```python
from build123d import *

# Parameters (mm, degrees)
SKETCH1_R           = 140
SKETCH1_R_2         = 5
SKETCH1_R_3         = 2.5
BOSS_EXTRUDE1_DEPTH = 2


with BuildPart() as part:
    # Sketch1 → Boss-Extrude1 (new body)
    with BuildSketch(Plane(origin=(0, 0, 0), x_dir=(1, 0, 0), z_dir=(0, 1, 0))):
        with Locations(Location((0, 0, 0), (0, 0, 270))):
            Circle(SKETCH1_R)
        with Locations(Location((-99.592921435, 57.5, 0), (0, 0, 270))):
            Circle(SKETCH1_R_2, mode=Mode.SUBTRACT)
        with Locations(Location((-57.5, 99.592921435, 0), (0, 0, 270))):
            Circle(SKETCH1_R_2, mode=Mode.SUBTRACT)
        with Locations(Location((57.5, 99.592921435, 0), (0, 0, 90))):
            Circle(SKETCH1_R_2, mode=Mode.SUBTRACT)
        with Locations(Location((99.592921435, 57.5, 0), (0, 0, 90))):
            Circle(SKETCH1_R_2, mode=Mode.SUBTRACT)
        with Locations(Location((99.592921435, -57.5, 0), (0, 0, 270))):
            Circle(SKETCH1_R_2, mode=Mode.SUBTRACT)
        with Locations(Location((57.5, -99.592921435, 0), (0, 0, 270))):
            Circle(SKETCH1_R_2, mode=Mode.SUBTRACT)
        with Locations(Location((-57.5, -99.592921435, 0), (0, 0, 90))):
            Circle(SKETCH1_R_2, mode=Mode.SUBTRACT)
        with Locations(Location((-99.592921435, -57.5, 0), (0, 0, 90))):
            Circle(SKETCH1_R_2, mode=Mode.SUBTRACT)
        with Locations(Location((0, 115, 0), (0, 0, 270))):
            Circle(SKETCH1_R_2, mode=Mode.SUBTRACT)
        with Locations(Location((0, -115, 0), (0, 0, 90))):
            Circle(SKETCH1_R_2, mode=Mode.SUBTRACT)
        with Locations(Location((-115, 0, 0), (0, 0, 270))):
            Circle(SKETCH1_R_2, mode=Mode.SUBTRACT)
        with Locations(Location((115, 0, 0), (0, 0, 90))):
            Circle(SKETCH1_R_2, mode=Mode.SUBTRACT)
        with Locations(Location((-10.352761804, 38.637033052, 0), (0, 0, 270))):
            Circle(SKETCH1_R_3, mode=Mode.SUBTRACT)
        with Locations(Location((-28.284271247, 28.284271247, 0), (0, 0, 270))):
            Circle(SKETCH1_R_3, mode=Mode.SUBTRACT)
        with Locations(Location((-38.637033052, 10.352761804, 0), (0, 0, 270))):
            Circle(SKETCH1_R_3, mode=Mode.SUBTRACT)
        with Locations(Location((-38.637033052, -10.352761804, 0), (0, 0, 270))):
            Circle(SKETCH1_R_3, mode=Mode.SUBTRACT)
        with Locations(Location((38.637033052, -10.352761804, 0), (0, 0, 90))):
            Circle(SKETCH1_R_3, mode=Mode.SUBTRACT)
        with Locations(Location((38.637033052, 10.352761804, 0), (0, 0, 90))):
            Circle(SKETCH1_R_3, mode=Mode.SUBTRACT)
        with Locations(Location((28.284271247, 28.284271247, 0), (0, 0, 90))):
            Circle(SKETCH1_R_3, mode=Mode.SUBTRACT)
        with Locations(Location((10.352761804, 38.637033052, 0), (0, 0, 90))):
            Circle(SKETCH1_R_3, mode=Mode.SUBTRACT)
        with Locations(Location((28.284271247, -28.284271247, 0), (0, 0, 270))):
            Circle(SKETCH1_R_3, mode=Mode.SUBTRACT)
        with Locations(Location((-28.284271247, -28.284271247, 0), (0, 0, 90))):
            Circle(SKETCH1_R_3, mode=Mode.SUBTRACT)
        with Locations(Location((10.352761804, -38.637033052, 0), (0, 0, 270))):
            Circle(SKETCH1_R_3, mode=Mode.SUBTRACT)
        with Locations(Location((-10.352761804, -38.637033052, 0), (0, 0, 90))):
            Circle(SKETCH1_R_3, mode=Mode.SUBTRACT)
    extrude(amount=BOSS_EXTRUDE1_DEPTH)


solid = part.part
```
The listing builds one solid part. Answer for the finished solid, in the listing's coordinates (mm). Round coordinates to 2 decimals unless told otherwise and drop trailing zeros. Loops run counter-clockwise (first coordinate to the right, second up) from the corner with the lowest first, then second, coordinate; pieces in that order, holes last. Notation, with made-up numbers: (-28, -19.5) - (3, -19.5) arc R15 cw to (3, -12.5) - close; hole circle Ø7 at (11.25, 19.5). An arc over 180 degrees is marked (long way). Use one line per item in the form item = value. Start each with the question number.
1. For a pull along X with two mould halves and no side action, classify faces 1 (the face through (2, 2, -2)), 2 (the face through (-85.19, 0.99, -111.1)), 3 (the face through (-96.214, 0.986, -61.185)) as pulls with the +X half, pulls with the -X half, needs draft (parallel to the pull), parting line crosses it, or undercut.
2. The part is cut by section C-C on z = -115. Determine the outline of the cut face in (x, y), then the cut area to 3 significant figures.
3. Consider line 1 (X direction, y = 0.55, z = 0); line 2 (X direction, y = 1.7, z = -104); line 3 (Z direction, x = -100.5, y = 1.15). Determine where each line is inside the solid, lowest interval first. Write a range as [from, to].
4. The part is cut by section B-B on x = 0. Determine the outline of the cut face in (y, z).
5. The part is cut by section A-A on z = 0. Determine the outline of the cut face in (x, y), then the cut area to 3 significant figures.
6. The part is cut by section D-D on x = 115. Determine the outline of the cut face in (y, z), then the cut area to 3 significant figures.
Geometry check:
q1.face_1 = needs draft
q1.face_2 = parting line crosses it
q1.face_3 = undercut
q2.outline = (-79.84, 0) - (-5, 0) - (-5, 2) - (-79.84, 2) - close; (5, 0) - (79.84, 0) - (79.84, 2) - (5, 2) - close
q2.area = 299 mm^2
q3.line_1 = [-140, -120], [-110, 110], [120, 140]
q3.line_2 = [-93.72, -59.86], [-55.14, 55.14], [59.86, 93.72]
q3.line_3 = [-97.47, -62.42], [-52.58, 52.58], [62.42, 97.47]
q4.outline = (0, -140) - (2, -140) - (2, -120) - (0, -120) - close; (0, -110) - (2, -110) - (2, 110) - (0, 110) - close; (0, 120) - (2, 120) - (2, 140) - (0, 140) - close
q5.outline = (-140, 0) - (-120, 0) - (-120, 2) - (-140, 2) - close; (-110, 0) - (110, 0) - (110, 2) - (-110, 2) - close; (120, 0) - (140, 0) - (140, 2) - (120, 2) - close
q5.area = 520 mm^2
q6.outline = (0, -79.84) - (2, -79.84) - (2, -5) - (0, -5) - close; (0, 5) - (2, 5) - (2, 79.84) - (0, 79.84) - close
q6.area = 299 mm^2
